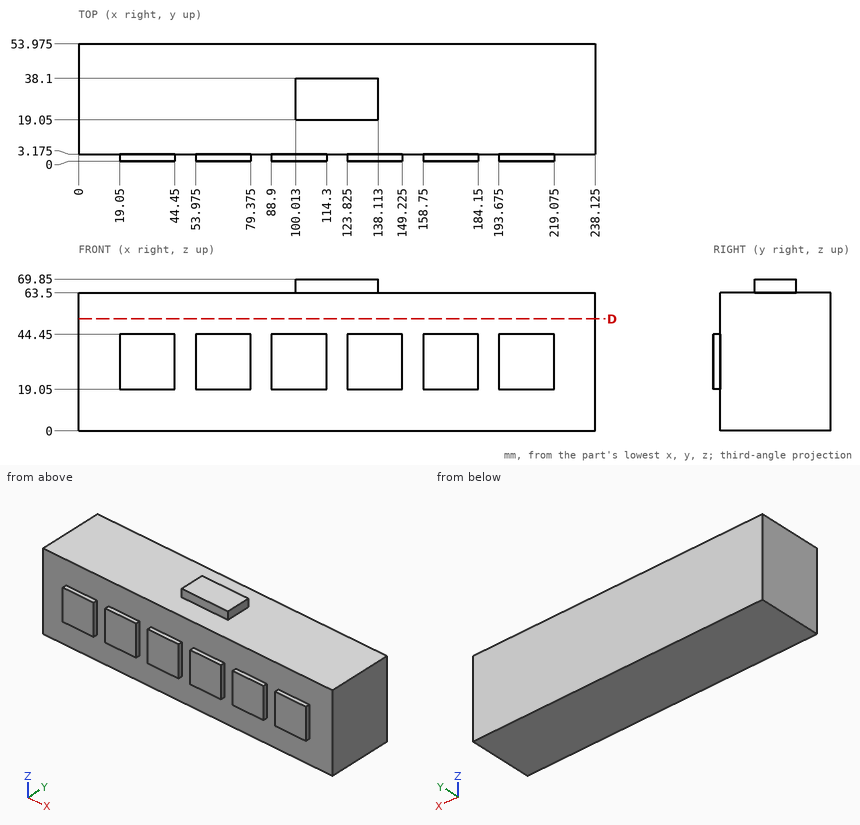
Study the drawing (mm; zero at the part's minimum x, y, z) and answer. Round coordinates to 2 decimals unless told otherwise and drop trailing zeros. Write each loop counter-clockwise with the first axis right and the second up, starting at its lowest first coordinate (ties: lowest second). Pieces come first, ordered by that corner, then holes.
1) Given pin 1 Ø1 at (y, z) = (2, 28.5) entering from -X; pin 2 Ø1.6 at (x, y) = (108, 1) entering from -Z; pin 3 Ø1 at (x, y) = (156.5, 45) entering from +Z, each flat-ended and moving along its own axis, determine where each tip first touches the part or whether it passes through.
2) A cutting plane is placed at D-D (z = 51.5). Give the vertices of the cut face in (x, y) (1 decimal).
3) Straight lines are drawn through the part: line 1 (Y direction, x = 187.5, z = 61) (1 decimal); line 2 (Z direction, x = 147.5, y = 25.5). For each, find the intervals that lie inside material, in ascending order.
Completed:
1. pin 1: stops at x = 19.05
1. pin 2: stops at z = 19.05
1. pin 3: stops at z = 63.5
2. outline: (0, 3.2) - (238.1, 3.2) - (238.1, 54) - (0, 54) - close
3. line 1: y = 3.2 to 54
3. line 2: z = 0 to 63.5
